from build123d import *

# Parameters (mm, degrees)
SKETCH1_W           = 25
SKETCH1_H           = 25
BOSS_EXTRUDE2_DEPTH = 10
SKETCH2_R           = 5.05
CUT_EXTRUDE1_DEPTH  = 26
SKETCH3_R           = 1.625
CUT_EXTRUDE2_DEPTH  = 11
SKETCH4_W           = 7.45
SKETCH4_H           = 25
CUT_EXTRUDE3_DEPTH  = 1


with BuildPart() as part:
    # Sketch1 → Boss-Extrude2 (new body)
    with BuildSketch(Plane.XY):
        Rectangle(SKETCH1_W, SKETCH1_H)
    extrude(amount=BOSS_EXTRUDE2_DEPTH)

    # Sketch2 → Cut-Extrude1 (cut, through all)
    with BuildSketch(Plane(origin=(0, 12.5, 0), x_dir=(1, 0, 0), z_dir=(0, 1, 0))):
        Circle(SKETCH2_R)
    extrude(amount=-CUT_EXTRUDE1_DEPTH, mode=Mode.SUBTRACT)

    # Sketch3 → Cut-Extrude2 (cut, through all)
    with BuildSketch(Plane.XY.offset(10)):
        with Locations((-8.964466094, 8.964466094)):
            Circle(SKETCH3_R)
        with Locations((8.964466094, 8.964466094)):
            Circle(SKETCH3_R)
        with Locations((8.964466094, -8.964466094)):
            Circle(SKETCH3_R)
        with Locations((-8.964466094, -8.964466094)):
            Circle(SKETCH3_R)
    extrude(amount=-CUT_EXTRUDE2_DEPTH, mode=Mode.SUBTRACT)

    # Sketch4 → Cut-Extrude3 (cut)
    with BuildSketch(Plane(origin=(0, 0, 0), x_dir=(-1, 0, 0), z_dir=(0, 0, -1))):
        with Locations((-8.775, 0)):
            Rectangle(SKETCH4_W, SKETCH4_H)
        with Locations((8.775, 0)):
            Rectangle(SKETCH4_W, SKETCH4_H)
    extrude(amount=-CUT_EXTRUDE3_DEPTH, mode=Mode.SUBTRACT)


solid = part.part
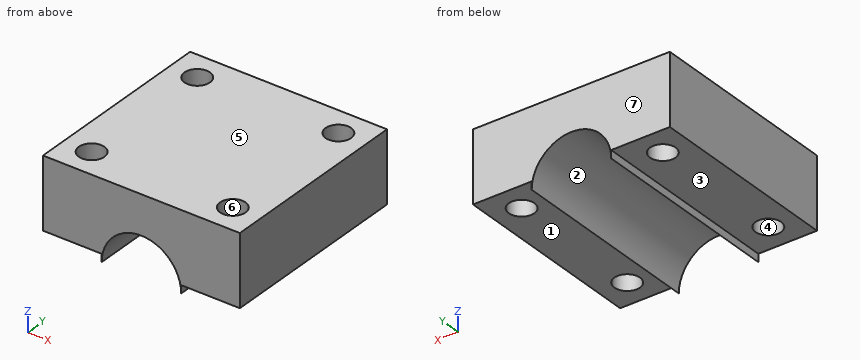
Can you work these out from the model? Positions are in its coordinate system, mm. Face numbers are marked on the shaded views. A direction names the side the tool comes from. Coordinates: 2 decimals unless noted, no trailing zeros. Write each loop counter-clockwise with the first axis right and the second up, starting at its lowest first coordinate (ties: lowest second). Pieces come first, ordered by that corner, then holes.
Q1. Imagine slicing it at B-B, the plane y = 3.75. List the corners of the cut face in (x, z) for me.
Results found:
outline: (-12.5, 1) - (-5.05, 1) - (-5.05, 0) arc R5.05 cw to (5.05, 0) - (5.05, 1) - (12.5, 1) - (12.5, 10) - (-12.5, 10) - close
Q2. If we mould it in two halves opening along Y, with no side actions, what happens to the marked faces 4, 5, 6 and 7? For each: +Y half, -Y half, draft (parallel to the pull), parting line (faces both ways), or undercut.
Results found:
face 4: undercut
face 5: draft
face 6: undercut
face 7: +Y half
Q3. Which directions (+Z, -Z, +X, -X, +Y, -Y) give clear straight access to the entire face, cutting with the end or side of a thin tool? Please do the marked faces 1, 2 and 3.
Results found:
face 1: -Z, +X, +Y, -Y
face 2: -Z, +Y, -Y
face 3: -Z, -X, +Y, -Y
Q4. Imagine slicing it at C-C, the plane x = 8.25. List the corners of the cut face in (y, z) for me, plus the area to 3 significant figures.
Results found:
outline: (-12.5, 1) - (-10.42, 1) - (-10.42, 10) - (-12.5, 10) - close; (-7.5, 1) - (7.5, 1) - (7.5, 10) - (-7.5, 10) - close; (10.42, 1) - (12.5, 1) - (12.5, 10) - (10.42, 10) - close
area: 172 mm2
Q5. Imagine slicing it at D-D, the plane z = 9.25. List the corners of the cut face in (x, y) for me (3 decimals).
Results found:
outline: (-12.5, -12.5) - (12.5, -12.5) - (12.5, 12.5) - (-12.5, 12.5) - close; hole circle Ø3.25 at (-8.964, -8.964); hole circle Ø3.25 at (-8.964, 8.964); hole circle Ø3.25 at (8.964, -8.964); hole circle Ø3.25 at (8.964, 8.964)
Q6. Imagine slicing it at A-A, the plane z = 1.75. List the corners of the cut face in (x, y) for me (3 decimals).
Results found:
outline: (-12.5, -12.5) - (-4.737, -12.5) - (-4.737, 12.5) - (-12.5, 12.5) - close; (4.737, -12.5) - (12.5, -12.5) - (12.5, 12.5) - (4.737, 12.5) - close; hole circle Ø3.25 at (-8.964, -8.964); hole circle Ø3.25 at (-8.964, 8.964); hole circle Ø3.25 at (8.964, -8.964); hole circle Ø3.25 at (8.964, 8.964)
Q7. For P1, Ø2, axis at x = -9, y = -2.5, coming from the -Z side; P2, Ø0.5, axis at y = 5.5, z = 0.5, coming from the -X side; P3, Ø0.8, axis at y = -2, z = 0.5, coming from the +X side, each with a flat end and sliding along its axis, tell me the tip position at first contact or that it passes through.
Results found:
P1: stops at z = 1
P2: stops at x = -5.05
P3: stops at x = 5.05
Q8. Please list where these lines run through material, in increasing order: L1, parallel to X at y = 9.5, z = 9.75; L2, parallel to Y at x = 8.75, z = 9.25; L3, parallel to X at y = 7.5, z = 3.
Results found:
L1: x = -12.5 to -10.5, -7.43 to 7.43, 10.5 to 12.5
L2: y = -12.5 to -10.58, -7.35 to 7.35, 10.58 to 12.5
L3: x = -12.5 to -9.67, -8.26 to -4.06, 4.06 to 8.26, 9.67 to 12.5
